```python
from build123d import *

# Parameters (mm, degrees)
SKETCH_W              = 20
SKETCH_H              = 28
PAD_DEPTH             = 28
SKETCH001_W           = 14
SKETCH001_H           = 24
POCKET_DEPTH          = 24
POCKET001_DEPTH       = 20.001
POCKET002_DEPTH       = 92.725292
POLARPATTERN_COUNT    = 2
POLARPATTERN_ANGLE    = 90
PAD001_DEPTH          = 2
POLARPATTERN001_COUNT = 2
POLARPATTERN001_ANGLE = 90


with BuildPart() as part:
    # Sketch → Pad (new body)
    with BuildSketch(Plane.XZ):
        with Locations((0, 14)):
            Rectangle(SKETCH_W, SKETCH_H)
    extrude(amount=PAD_DEPTH)

    # Sketch001 (on Face6 of Pad) → Pocket (cut)
    with BuildSketch(Plane.XZ.offset(28)):
        with Locations((0, 16)):
            Rectangle(SKETCH001_W, SKETCH001_H)
    extrude(amount=-POCKET_DEPTH, mode=Mode.SUBTRACT)

    # Sketch002 (on Face3 of Pocket) → Pocket001 (cut, through all)
    with BuildSketch(Plane(origin=(10, 0, 0), x_dir=(0, 0, 1), z_dir=(1, 0, 0))):
        Polygon((6.5, 28), (6.5, 21.5), (21.5, 6.5), (28, 6.5), (28, 28), align=None)
    extrude(amount=-POCKET001_DEPTH, mode=Mode.SUBTRACT)

    # Sketch003 (on Face16 of Pocket001) → Pocket002 (cut, through all)
    with BuildSketch(Plane.XZ.offset(4)):
        with BuildLine():
            ThreePointArc((3.25, 15.5), (0, 18.75), (-3.25, 15.5))
            Line((-3.25, 15.5), (-3.25, 12.5))
            ThreePointArc((-3.25, 12.5), (0, 9.25), (3.25, 12.5))
            Line((3.25, 15.5), (3.25, 12.5))
        make_face()
    pocket002 = extrude(amount=-POCKET002_DEPTH, mode=Mode.SUBTRACT)

    # PolarPattern: Pocket002 ×2 about axis
    polarpattern_axis = Axis((0, 0, 0), (1, 0, 0))
    for i in range(1, POLARPATTERN_COUNT):
        add(pocket002.rotate(polarpattern_axis, i * POLARPATTERN_ANGLE / (POLARPATTERN_COUNT - 1)), mode=Mode.SUBTRACT)

    # Sketch004 (on Face3 of PolarPattern) → Pad001 (join, symmetric)
    with BuildSketch(Plane(origin=(0, 0, 0), x_dir=(1, 0, 0), z_dir=(0, 1, 0))):
        with BuildLine():
            ThreePointArc((-1.9, -2), (-2.9, -3), (-1.9, -4))
            Line((-1.9, -4), (1.9, -4))
            ThreePointArc((1.9, -4), (2.9, -3), (1.9, -2))
            Line((-1.9, -2), (1.9, -2))
        make_face()
        with BuildLine():
            ThreePointArc((-1.9, -24), (-2.9, -25), (-1.9, -26))
            Line((-1.9, -26), (1.9, -26))
            ThreePointArc((1.9, -26), (2.9, -25), (1.9, -24))
            Line((-1.9, -24), (1.9, -24))
        make_face()
    pad001 = extrude(amount=PAD001_DEPTH, both=True)

    # PolarPattern001: Pad001 ×2 about axis
    polarpattern001_axis = Axis((0, 0, 0), (1, 0, 0))
    for i in range(1, POLARPATTERN001_COUNT):
        add(pad001.rotate(polarpattern001_axis, i * POLARPATTERN001_ANGLE / (POLARPATTERN001_COUNT - 1)))


solid = part.part
```
CAD build for the part. Positions are in the model's coordinates, mm. A direction names the side the tool comes from. Round coordinates to 2 decimals unless told otherwise and drop trailing zeros. Order: outer loops, then holes, each group sorted by start corner. A loop starts at its lowest first (then second) coordinate and runs counter-clockwise, first axis right, second up.
Q1. Slice it at B-B (x = 0). State how many separate pieces and enclosed holes the cut face has, and give its area (3 significant figures).
Q2. Wall check: L1, parallel to X at y = -19, z = 8.5; L2, parallel to Y at x = 7.25, z = 24.5; L3, parallel to Z at x = -3.25, y = -8.25. Give the ranges that are in metal, low to high.
Q3. Drop flat-ended pins along their axis: pin 1 (10 mm diameter, centred on x = 6, z = 20, fed in from +Y); pin 2 (2.5 mm diameter, centred on x = -9, z = 25.5, fed in from -Y); pin 3 (0.6 mm diameter, centred on x = 0.5, z = -1, fed in from +Y). Give the stop position or say it passes through.
Q4. Slice it at D-D (y = -25). Write the cut outline in (x, z).
Q5. Which spindle directions (+Z, -Z, +X, -X, +Y, -Y) get a long thin tool onto all of the face, cutting with end or side? Do faces 4 (the cylindrical face through (-2.9, 1, 3)), 5 (the flat face through (9, -6.5, 25)), 6 (the cylindrical face through (0.07, -18.75, 1.97)), 7 (the flat face through (0, 1, 26)). Say none if no direction does.
Q6. Two-plate mould, pull along Y, no slides. Class faces 1 (the flat face through (0, 2, 25)), 2 (the flat face through (0, 1, 4)), 3 (the cylindrical face through (-0.07, -9.25, 1.97)): pulls with the +Y half, pulls with the -Y half, needs draft (parallel to the pull), parting line crosses it, or undercut.
Q7. Slice it at A-A (y = -3). Write the cut outline in (x, z), and give its area (3 significant figures).
Q8. Slice it at C-C (z = 17.5). Write the cut outline in (x, y).
Results below:
1. separate pieces: 3
1. enclosed holes: 0
1. area: 148 mm2
2. L1: x = -10 to -7, 7 to 10
2. L2: y = -6.5 to 0
2. L3: z = 0 to 4
3. pin 1: stops at y = 0
3. pin 2: stops at y = -6.5
3. pin 3: stops at y = -2
4. outline: (-10, 0) - (-2.9, 0) - (-2.9, -2) - (2.9, -2) - (2.9, 0) - (10, 0) - (10, 6.5) - (7, 6.5) - (7, 4) - (-7, 4) - (-7, 6.5) - (-10, 6.5) - close
5. face 4: -X, +Y
5. face 5: +Z, +X, -X, -Y
5. face 6: +Z, -Z
5. face 7: +Z, +X, -X, +Y
6. face 1: pulls with the +Y half
6. face 2: needs draft
6. face 3: undercut
7. outline: (-10, 0) - (-2.9, 0) - (-2.9, -2) - (2.9, -2) - (2.9, 0) - (10, 0) - (10, 28) - (-10, 28) - close; hole (-3.25, 12.5) arc R3.25 ccw to (3.25, 12.5) - (3.25, 15.5) arc R3.25 ccw to (-3.25, 15.5) - close
7. area: 519 mm2
8. outline: (-10, -10.5) - (-7, -10.5) - (-7, -4) - (-2.56, -4) - (-2.56, 0) - (-10, 0) - close; (2.56, -4) - (7, -4) - (7, -10.5) - (10, -10.5) - (10, 0) - (2.56, 0) - close
